CAD build for the part. Positions are in the model's coordinates, mm. Give positions to 0.01 mm unless a question says otherwise; leave off trailing zeros. Order: outer loops, then holes, each group sorted by start corner. A loop starts at its lowest first (then second) coordinate and runs counter-clockwise, first axis right, second up.
```python
from build123d import *

# Parameters (mm, degrees)
SKETCH1_W                   = 25.4
SKETCH1_H                   = 12.7
BOSS_EXTRUDE1_DEPTH         = 6.35
F_3_16_0_1875_DOWEL_HOLE1_D = 4.7625
SKETCH6_R                   = 3.175
CUT_EXTRUDE1_DEPTH          = 6.35


with BuildPart() as part:
    # Sketch1 → Boss-Extrude1 (new, symmetric)
    with BuildSketch(Plane.XY):
        with Locations((12.7, 6.35)):
            Rectangle(SKETCH1_W, SKETCH1_H)
    extrude(amount=BOSS_EXTRUDE1_DEPTH, both=True)

    # 3/16 (0.1875) Dowel Hole1 (through all)
    with Locations(Plane(origin=(13.97, 12.7, -1.905), x_dir=(0, 0, 1), z_dir=(0, 1, 0))):
        with Locations((0, 0), (0, -10.0076)):
            Hole(F_3_16_0_1875_DOWEL_HOLE1_D / 2)

    # Sketch6 → Cut-Extrude1 (cut)
    with BuildSketch(Plane(origin=(25.4, 0, 0), x_dir=(0, 0, -1), z_dir=(1, 0, 0))):
        with Locations((0, 6.35)):
            Circle(SKETCH6_R)
    extrude(amount=-CUT_EXTRUDE1_DEPTH, mode=Mode.SUBTRACT)


solid = part.part
```
Item 1: Wall check: L1, parallel to X at y = 7, z = -2; L2, parallel to X at y = 3.5, z = -2.5; L3, parallel to Y at x = 22.25, z = 0 (3 decimals). Give the ranges that are in metal, low to high.
Item 2: Slice it at B-B (x = 3.25). Give the cut face in (y, z).
Item 3: Two-plate mould, pull along Y, no slides. Class faces 1 (the face through (19.05, 6, 0)), 2 (the face through (13, 0, 2)), 3 (the face through (13, 6, 6.35)), 4 (the face through (22.269, 9.027, -1.707)): released by +Y, released by -Y, zero draft, split by the parting line, or undercut.
Item 4: Slice it at A-A (z = -2.5). Give the cut face in (x, y).
Item 5: Slice it at C-C (x = 20). Give the cut face in (y, z) (3 decimals), and give its area (3 significant figures).
Item 6: Slice it at D-D (y = 6.35). State how many separate pieces and enclosed holes the cut face has, and give its area (3 significant figures).
Item 7: Drop flat-ended pins along their axis: pin 1 Ø4 at (y, z) = (7, 0.5) entering from +X; pin 2 Ø4 at (x, z) = (10, 0) entering from -Y. Give the stop position or say it passes through.
A:
1. L1: x = 0 to 1.58, 6.34 to 11.59, 16.35 to 19.05
1. L2: x = 0 to 1.66, 6.27 to 11.66, 16.28 to 25.4
1. L3: y = 0 to 3.175, 9.525 to 12.7
2. outline: (0, -6.35) - (12.7, -6.35) - (12.7, -4.18) - (0, -4.18) - close; (0, 0.37) - (12.7, 0.37) - (12.7, 6.35) - (0, 6.35) - close
3. face 1: undercut
3. face 2: released by -Y
3. face 3: zero draft
3. face 4: undercut
4. outline: (0, 0) - (1.66, 0) - (1.66, 12.7) - (0, 12.7) - close; (6.27, 0) - (11.66, 0) - (11.66, 12.7) - (6.27, 12.7) - close; (16.28, 0) - (25.4, 0) - (25.4, 4.39) - (19.05, 4.39) - (19.05, 8.31) - (25.4, 8.31) - (25.4, 12.7) - (16.28, 12.7) - close
5. outline: (0, -6.35) - (12.7, -6.35) - (12.7, 6.35) - (0, 6.35) - close; hole circle Ø6.35 at (6.35, 0)
5. area: 130 mm2
6. separate pieces: 1
6. enclosed holes: 2
6. area: 247 mm2
7. pin 1: stops at x = 19.05
7. pin 2: stops at y = 0
